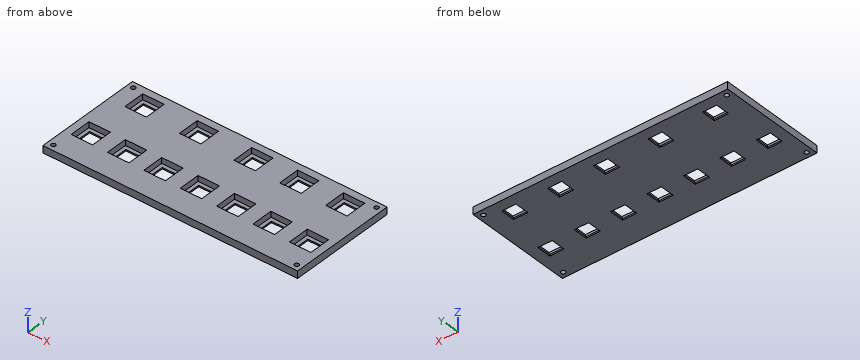
Autodesk Fusion 360 part; units mm, degrees
sketch "Sketch1" plane through (0, 0, 0) normal (0, 0, 1) x (1, 0, 0)
  line L0 (-23.9041, 0) -> (63.45, 0) construction
  line L1 (78.95, 0) -> (176.0959, 0) construction
  line L2 (-1.45, -20) -> (177.05, -20)
  line L3 (177.05, -20) -> (177.05, 55.5)
  line L4 (177.05, 55.5) -> (-1.45, 55.5)
  line L5 (-1.45, 55.5) -> (-1.45, -20)
  line L6 (6.3, 0) -> (16.3, 0)
  line L7 (16.3, 0) -> (16.3, 10)
  line L8 (16.3, 10) -> (6.3, 10)
  line L9 (6.3, 10) -> (6.3, 0)
  line L10 (31.8, 0) -> (41.8, 0)
  line L11 (41.8, 0) -> (41.8, 10)
  line L12 (41.8, 10) -> (31.8, 10)
  line L13 (31.8, 10) -> (31.8, 0)
  line L14 (57.3, 0) -> (67.3, 0)
  line L15 (67.3, 0) -> (67.3, 10)
  line L16 (67.3, 10) -> (57.3, 10)
  line L17 (57.3, 10) -> (57.3, 0)
  line L18 (82.8, 0) -> (92.8, 0)
  line L19 (92.8, 0) -> (92.8, 10)
  line L20 (92.8, 10) -> (82.8, 10)
  line L21 (82.8, 10) -> (82.8, 0)
  line L22 (108.3, 0) -> (118.3, 0)
  line L23 (118.3, 0) -> (118.3, 10)
  line L24 (118.3, 10) -> (108.3, 10)
  line L25 (108.3, 10) -> (108.3, 0)
  line L26 (133.8, 0) -> (143.8, 0)
  line L27 (143.8, 0) -> (143.8, 10)
  line L28 (143.8, 10) -> (133.8, 10)
  line L29 (133.8, 10) -> (133.8, 0)
  line L30 (159.3, 0) -> (169.3, 0)
  line L31 (169.3, 0) -> (169.3, 10)
  line L32 (169.3, 10) -> (159.3, 10)
  line L33 (159.3, 10) -> (159.3, 0)
  line L34 (12.45, 48) -> (22.45, 48)
  line L35 (22.45, 48) -> (22.45, 38)
  line L36 (22.45, 38) -> (12.45, 38)
  line L37 (12.45, 38) -> (12.45, 48)
  line L38 (50.65, 48) -> (60.65, 48)
  line L39 (60.65, 48) -> (60.65, 38)
  line L40 (60.65, 38) -> (50.65, 38)
  line L41 (50.65, 38) -> (50.65, 48)
  line L42 (88.85, 48) -> (98.85, 48)
  line L43 (98.85, 48) -> (98.85, 38)
  line L44 (98.85, 38) -> (88.85, 38)
  line L45 (88.85, 38) -> (88.85, 48)
  line L46 (121, 48) -> (131, 48)
  line L47 (131, 48) -> (131, 38)
  line L48 (131, 38) -> (121, 38)
  line L49 (121, 38) -> (121, 48)
  line L50 (153.15, 48) -> (163.15, 48)
  line L51 (163.15, 48) -> (163.15, 38)
  line L52 (163.15, 38) -> (153.15, 38)
  line L53 (153.15, 38) -> (153.15, 48)
  line L54 (9.95, 50.5) -> (24.95, 50.5)
  line L55 (24.95, 50.5) -> (24.95, 35.5)
  line L56 (24.95, 35.5) -> (9.95, 35.5)
  line L57 (9.95, 35.5) -> (9.95, 50.5)
  line L58 (9.95, 50.5) -> (24.95, 35.5) construction
  line L59 (24.95, 50.5) -> (9.95, 35.5) construction
  line L60 (48.15, 50.5) -> (63.15, 50.5)
  line L61 (63.15, 50.5) -> (63.15, 35.5)
  line L62 (63.15, 35.5) -> (48.15, 35.5)
  line L63 (48.15, 35.5) -> (48.15, 50.5)
  line L64 (48.15, 50.5) -> (63.15, 35.5) construction
  line L65 (63.15, 50.5) -> (48.15, 35.5) construction
  line L66 (86.35, 50.5) -> (101.35, 50.5)
  line L67 (101.35, 50.5) -> (101.35, 35.5)
  line L68 (101.35, 35.5) -> (86.35, 35.5)
  line L69 (86.35, 35.5) -> (86.35, 50.5)
  line L70 (86.35, 50.5) -> (101.35, 35.5) construction
  line L71 (101.35, 50.5) -> (86.35, 35.5) construction
  line L72 (118.5, 50.5) -> (133.5, 50.5)
  line L73 (133.5, 50.5) -> (133.5, 35.5)
  line L74 (133.5, 35.5) -> (118.5, 35.5)
  line L75 (118.5, 35.5) -> (118.5, 50.5)
  line L76 (118.5, 50.5) -> (133.5, 35.5) construction
  line L77 (133.5, 50.5) -> (118.5, 35.5) construction
  line L78 (150.65, 50.5) -> (165.65, 50.5)
  line L79 (165.65, 50.5) -> (165.65, 35.5)
  line L80 (165.65, 35.5) -> (150.65, 35.5)
  line L81 (150.65, 35.5) -> (150.65, 50.5)
  line L82 (150.65, 50.5) -> (165.65, 35.5) construction
  line L83 (165.65, 50.5) -> (150.65, 35.5) construction
  line L84 (3.8, 12.5) -> (18.8, 12.5)
  line L85 (18.8, 12.5) -> (18.8, -2.5)
  line L86 (18.8, -2.5) -> (3.8, -2.5)
  line L87 (3.8, -2.5) -> (3.8, 12.5)
  line L88 (3.8, 12.5) -> (18.8, -2.5) construction
  line L89 (18.8, 12.5) -> (3.8, -2.5) construction
  line L90 (29.3, 12.5) -> (44.3, 12.5)
  line L91 (44.3, 12.5) -> (44.3, -2.5)
  line L92 (44.3, -2.5) -> (29.3, -2.5)
  line L93 (29.3, -2.5) -> (29.3, 12.5)
  line L94 (29.3, 12.5) -> (44.3, -2.5) construction
  line L95 (44.3, 12.5) -> (29.3, -2.5) construction
  line L96 (54.8, 12.5) -> (69.8, 12.5)
  line L97 (69.8, 12.5) -> (69.8, -2.5)
  line L98 (69.8, -2.5) -> (54.8, -2.5)
  line L99 (54.8, -2.5) -> (54.8, 12.5)
  line L100 (54.8, 12.5) -> (69.8, -2.5) construction
  line L101 (69.8, 12.5) -> (54.8, -2.5) construction
  line L102 (80.3, 12.5) -> (95.3, 12.5)
  line L103 (95.3, 12.5) -> (95.3, -2.5)
  line L104 (95.3, -2.5) -> (80.3, -2.5)
  line L105 (80.3, -2.5) -> (80.3, 12.5)
  line L106 (80.3, 12.5) -> (95.3, -2.5) construction
  line L107 (95.3, 12.5) -> (80.3, -2.5) construction
  line L108 (105.8, 12.5) -> (120.8, 12.5)
  line L109 (120.8, 12.5) -> (120.8, -2.5)
  line L110 (120.8, -2.5) -> (105.8, -2.5)
  line L111 (105.8, -2.5) -> (105.8, 12.5)
  line L112 (105.8, 12.5) -> (120.8, -2.5) construction
  line L113 (120.8, 12.5) -> (105.8, -2.5) construction
  line L114 (131.3, 12.5) -> (146.3, 12.5)
  line L115 (146.3, 12.5) -> (146.3, -2.5)
  line L116 (146.3, -2.5) -> (131.3, -2.5)
  line L117 (131.3, -2.5) -> (131.3, 12.5)
  line L118 (131.3, 12.5) -> (146.3, -2.5) construction
  line L119 (146.3, 12.5) -> (131.3, -2.5) construction
  line L120 (156.8, 12.5) -> (171.8, 12.5)
  line L121 (171.8, 12.5) -> (171.8, -2.5)
  line L122 (171.8, -2.5) -> (156.8, -2.5)
  line L123 (156.8, -2.5) -> (156.8, 12.5)
  line L124 (156.8, 12.5) -> (171.8, -2.5) construction
  line L125 (171.8, 12.5) -> (156.8, -2.5) construction
  circle A0 centre (2.55, 51.5) radius 1.5
  circle A1 centre (2.55, -16) radius 1.5
  circle A2 centre (173.05, -16) radius 1.5
  circle A3 centre (173.05, 51.5) radius 1.5
  point P0 (-11.7503, 0.5527)
  point P1 (17.45, 43)
  point P2 (55.65, 43)
  point P3 (93.85, 43)
  point P4 (126, 43)
  point P5 (158.15, 43)
  point P6 (11.3, 5)
  point P7 (36.8, 5)
  point P8 (62.3, 5)
  point P9 (87.8, 5)
  point P10 (113.3, 5)
  point P11 (138.8, 5)
  point P12 (164.3, 5)
  dimension "d77" = 200
  dimension "d86" = 75.5
  dimension "d89" = 10
  dimension "d90" = 10
  dimension "d91" = 20
  dimension "d92" = 7.75
  dimension "d93" = 10
  dimension "d94" = 10
  dimension "d95" = 10
  dimension "d96" = 10
  dimension "d99" = 10
  dimension "d100" = 10
  dimension "d101" = 15.5
  dimension "d102" = 15.5
  dimension "d104" = 15.5
  dimension "d105" = 10
  dimension "d106" = 10
  dimension "d107" = 15.5
  dimension "d108" = 10
  dimension "d109" = 10
  dimension "d110" = 15.5
  dimension "d111" = 10
  dimension "d112" = 10
  dimension "d113" = 15.5
  dimension "d114" = 10
  dimension "d115" = 10
  dimension "d116" = 13.9
  dimension "d117" = 7.5
  dimension "d118" = 10
  dimension "d119" = 10
  dimension "d120" = 7.5
  dimension "d121" = 28.2
  dimension "d122" = 10
  dimension "d123" = 10
  dimension "d124" = 28.2
  dimension "d125" = 7.5
  dimension "d126" = 10
  dimension "d127" = 10
  dimension "d128" = 22.15
  dimension "d129" = 7.5
  dimension "d130" = 10
  dimension "d131" = 10
  dimension "d132" = 22.15
  dimension "d133" = 7.5
  dimension "d134" = 15
  dimension "d135" = 15
  dimension "d136" = 15
  dimension "d137" = 15
  dimension "d138" = 15
  dimension "d139" = 15
  dimension "d140" = 15
  dimension "d141" = 15
  dimension "d142" = 15
  dimension "d143" = 15
  dimension "d144" = 15
  dimension "d145" = 15
  dimension "d146" = 15
  dimension "d147" = 15
  dimension "d148" = 15
  dimension "d149" = 15
  dimension "d150" = 15
  dimension "d151" = 15
  dimension "d152" = 15
  dimension "d153" = 15
  dimension "d154" = 15
  dimension "d155" = 15
  dimension "d156" = 15
  dimension "d157" = 15
  dimension "d158" = 3
  dimension "d159" = 4
  dimension "d160" = 4
  dimension "d161" = 3
  dimension "d162" = 4
  dimension "d163" = 4
  dimension "d164" = 3
  dimension "d165" = 4
  dimension "d166" = 4
  dimension "d167" = 3
  dimension "d168" = 4
  dimension "d169" = 4
  dimension "d174" = 2.5
  dimension "d175" = 2.5
  dimension "d176" = 2.5
  dimension "d177" = 2.5
  dimension "d178" = 2.5
  dimension "d179" = 2.5
  dimension "d182" = 5.25
  dimension "d183" = 2.5
  dimension "d184" = 2.5
  dimension "d185" = 2.5
  dimension "d186" = 2.5
  dimension "d187" = 2.5
  dimension "d188" = 2.5
  dimension "d189" = 2.5
  dimension "d190" = 2.5
  dimension "d191" = 2.5
  dimension "d192" = 2.5
  dimension "d193" = 2.5
extrude "Extrude1" add sketch "Sketch1" along normal blind 1 contours L54 L55 L56 L57 | L60 L61 L62 L63 | L66 L67 L68 L69 | L72 L73 L74 L75 | L78 L79 L80 L81 | L84 L85 L86 L87 | L90 L91 L92 L93 | L96 L97 L98 L99 | L102 L103 L104 L105 | L108 L109 L110 L111 | L114 L115 L116 L117 | L120 L121 L122 L123 makes body 1 at (140.4667, 11.6667, 0) makes body 2 at (89.4667, 11.6667, 0) makes body 3 at (12.9667, -1.6667, 0) makes body 4 at (35.1333, 11.6667, 0) makes body 5 at (95.5167, 36.3333, 0) makes body 6 at (151.4833, 41.3333, 0) makes body 7 at (119.3333, 41.3333, 0) makes body 8 at (60.6333, -1.6667, 0) makes body 9 at (24.1167, 44.6667, 0) makes body 10 at (57.3167, 49.6667, 0) makes body 11 at (114.9667, -1.6667, 0) makes body 12 at (162.6333, 11.6667, 0)
extrude "Extrude2" add sketch "Sketch1" along normal blind 5 contours L2 L3 L4 L5 bodies 1 2 3 4 5 6 7 8 9 10 11 12
Here's how the part is built. I have some questions about the finished solid (model axes, mm). Round coordinates to 2 decimals unless told otherwise and drop trailing zeros.
1. Will these pins go through, and if not, where does the flat tip stop? pin 1 (12 mm diameter, centred on x = 142.5, y = 31, fed in from -Z); pin 2 (4.5 mm diameter, centred on x = 14.5, y = 4.5, fed in from +Z).
Answers:
pin 1: stops at z = 0
pin 2: stops at z = 1
2. If I drill on probe 1 along Y at (x, z) = (2.55, 3.5); probe 2 along X at (y, z) = (44.5, 0.8); probe 3 along Y at (x, z) = (56, 3), over which ranges is the centre line in solid material (lowest first)?
Answers:
probe 1: y = -20 to -17.5, -14.5 to 50, 53 to 55.5
probe 2: x = -1.45 to 12.45, 22.45 to 50.65, 60.65 to 88.85, 98.85 to 121, 131 to 153.15, 163.15 to 177.05
probe 3: y = -20 to -2.5, 12.5 to 35.5, 50.5 to 55.5
3. Suppose I cut it at A-A, the plane z = 3.55. Give the number of separate pieces and of enclosed holes in the cut face, and give its area (3 significant figures).
Answers:
separate pieces: 1
enclosed holes: 16
area: 10,700 mm2
